Verification items for this drawing (mm, ordinates from the low corner). Round coordinates to 2 decimals unless told otherwise and drop trailing zeros. Order: outer loops, then holes, each group sorted by start corner. A loop starts at its lowest first (then second) coordinate and runs counter-clockwise, first axis right, second up.
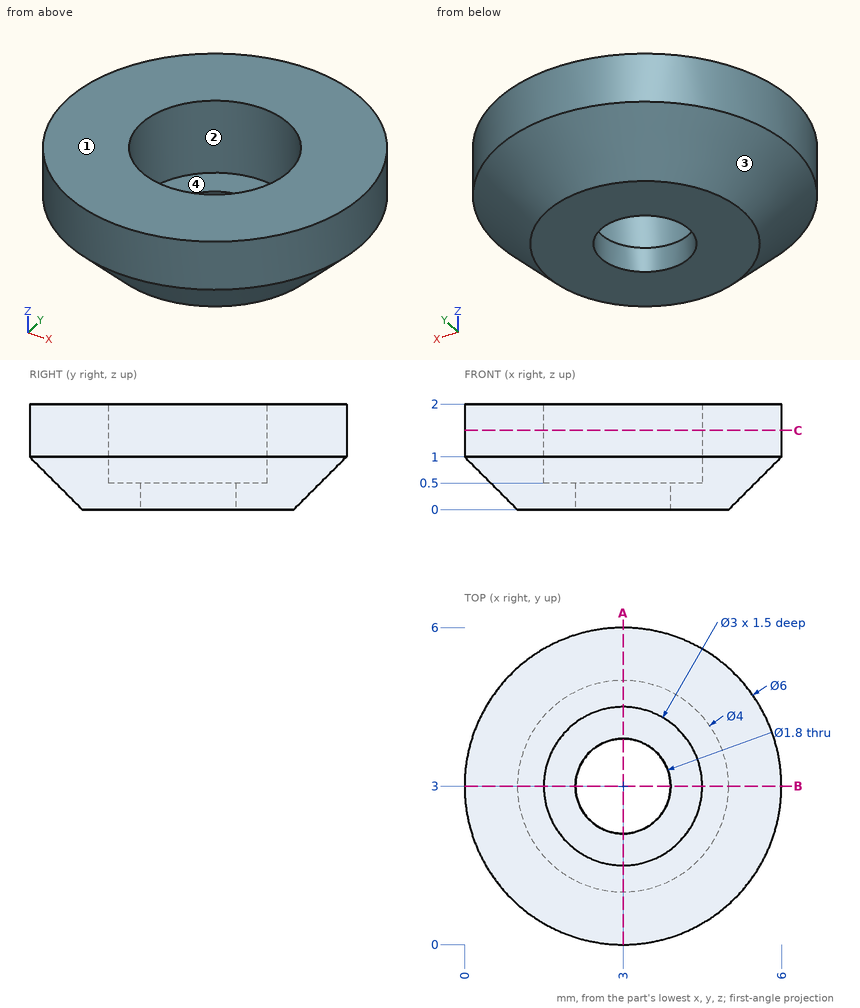
Item 1: Sectioned sample at C-C (z = 1.5). Record the cut outline in (x, y).
Answer:
outline: circle Ø6 at (3, 3); hole circle Ø3 at (3, 3)
Item 2: Go/stop test with flat-tipped pins: P1, Ø1.4, axis at x = 3, y = 3, coming from the -Z side; P2, Ø1.5, axis at x = 3.5, y = 3, coming from the +Z side. Record where each tip stops, or that it passes through.
Answer:
P1: passes through
P2: stops at z = 0.5
Item 3: Sectioned sample at A-A (x = 3). Record the cut outline in (y, z).
Answer:
outline: (0, 1) - (1, 0) - (2.1, 0) - (2.1, 0.5) - (1.5, 0.5) - (1.5, 2) - (0, 2) - close; (3.9, 0) - (5, 0) - (6, 1) - (6, 2) - (4.5, 2) - (4.5, 0.5) - (3.9, 0.5) - close
Item 4: Scan lines: line 1 along Y through (x, z) = (3, 1.3); line 2 along Z through (x, y) = (4.1, 2.8); line 3 along Y through (x, z) = (2.6, 0.7). Record each from-to range of solid material in increasing order.
Answer:
line 1: y = 0 to 1.5, 4.5 to 6
line 2: z = 0 to 0.5
line 3: y = 0.33 to 1.55, 4.45 to 5.67
Item 5: Release check for a two-part mould opening along Y. For the marked faces 1, 2, 3 and 4 record: released by +Y, released by -Y, zero draft, split by the parting line, or undercut.
Answer:
face 1: zero draft
face 2: undercut
face 3: split by the parting line
face 4: undercut
